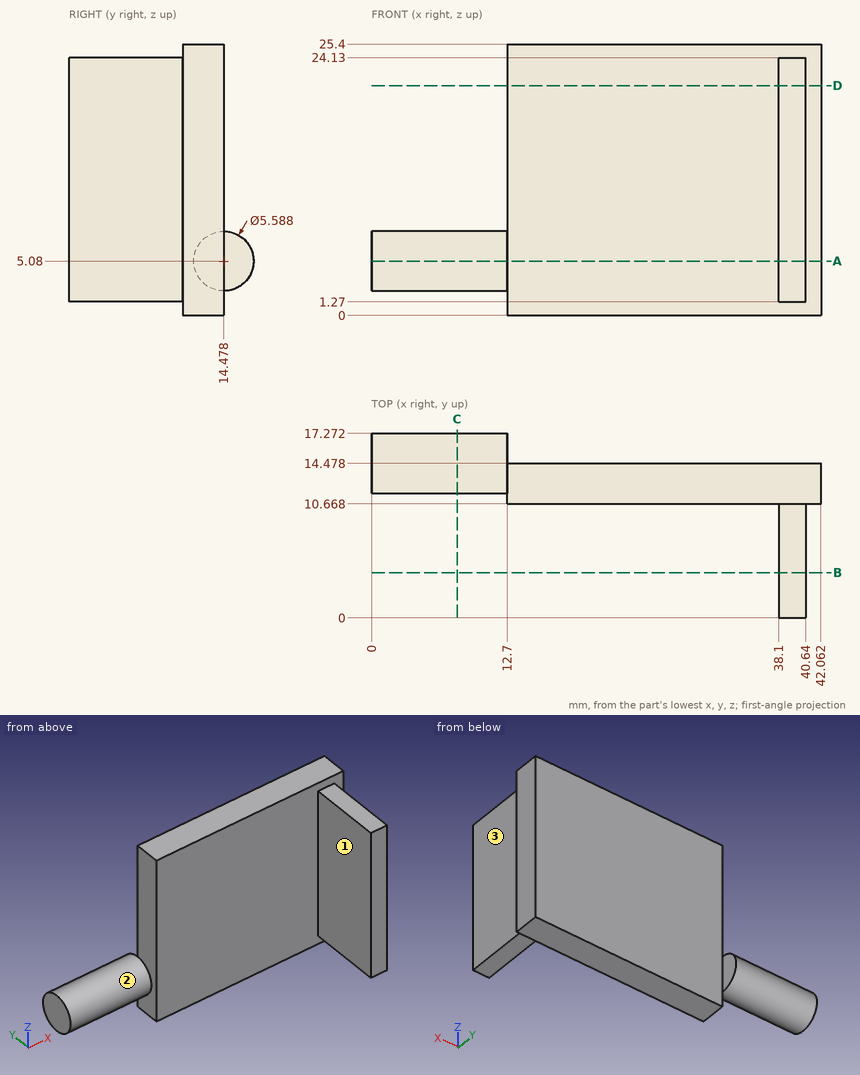
Job drawing, mm, ordinate dimensions from the low corner. One solid piece. A direction names the side the tool comes from. Give positions to 0.01 mm unless a question says otherwise; leave off trailing zeros. Loops run counter-clockwise (first coordinate to the right, second up) from the corner with the lowest first, then second, coordinate; pieces in that order, holes last. Notation, with made-up numbers: M -13.75,-31.5 L -4.75,-31.5 A32 cw -4.75,-0.5 Z; hole C 9,74 d2. An arc over 180 degrees is marked long. Return JSON: item names as keys, results as strings.
1) 3-axis set-ups, long thin cutter, end or side, ignore diameter. For the marked faces 1, 2 and 3: which of +Z, -Z, +X, -X, +Y, -Y reach the whole face in a straight line?
Calculated:
{"face 1": "+Z, -Z, -X, -Y", "face 2": "-X", "face 3": "+Z, -Z, +X, -Y"}
2) Flat gauge pins, fed straight in: pin 1 Ø0.8 at (y, z) = (15.5, 6.5) entering from +X; pin 2 Ø8 at (y, z) = (14.5, 3) entering from +X; pin 3 Ø8.5 at (y, z) = (4.5, 17.5) entering from -X; pin 4 Ø4 at (y, z) = (12.5, 11.5) entering from -X. Where does each tip first touch, or does it go through?
Calculated:
{"pin 1": "stops at x = 12.7", "pin 2": "stops at x = 42.06", "pin 3": "stops at x = 38.1", "pin 4": "stops at x = 12.7"}
3) Saw through at A-A, the plane z = 5.08. List the corners of the cut face in (x, y).
Calculated:
{"outline": "M 0,11.68 L 12.7,11.68 L 12.7,10.67 L 38.1,10.67 L 38.1,0 L 40.64,0 L 40.64,10.67 L 42.06,10.67 L 42.06,14.48 L 12.7,14.48 L 12.7,17.27 L 0,17.27 Z"}
4) Saw through at C-C, the plane x = 8. List the corners of the cut face in (y, z).
Calculated:
{"outline": "C 14.48,5.08 d5.59"}
5) Saw through at D-D, the plane z = 21.5. List the corners of the cut face in (x, y).
Calculated:
{"outline": "M 12.7,10.67 L 38.1,10.67 L 38.1,0 L 40.64,0 L 40.64,10.67 L 42.06,10.67 L 42.06,14.48 L 12.7,14.48 Z"}
6) Saw through at B-B, the plane y = 4.25. List the corners of the cut face in (x, z).
Calculated:
{"outline": "M 38.1,1.27 L 40.64,1.27 L 40.64,24.13 L 38.1,24.13 Z"}
7) Drill centre lines: line 1 (X direction, y = 10.5, z = 16.25); line 2 (Y direction, x = 13, z = 14); line 3 (Y direction, x = 2, z = 5) (1 decimal). Where is each one in solid material? Low to high.
Calculated:
{"line 1": "x = 38.1 to 40.64", "line 2": "y = 10.67 to 14.48", "line 3": "y = 11.7 to 17.3"}
